```python
from build123d import *

# Parameters (mm, degrees)
SKETCH2_R           = 75
SKETCH2_R_2         = 59
SKETCH2_R_3         = 46.992946112
BOSS_EXTRUDE1_DEPTH = 6
SKETCH4_R           = 2.5
CUT_EXTRUDE1_DEPTH  = 8
SKETCH5_R           = 1.9
CUT_EXTRUDE2_DEPTH  = 8
SKETCH8_R           = 25
CUT_EXTRUDE4_DEPTH  = 2


with BuildPart() as part:
    # Sketch1 → Revolve1 (revolve)
    with BuildSketch(Plane(origin=(0, 0, 0), x_dir=(-1, 0, 0), z_dir=(0, 0, -1)), mode=Mode.PRIVATE) as revolve1_sk:
        with BuildLine():
            Line((-59, 0.8724), (-47, 0.8724))
            ThreePointArc((-47, 0.8724), (-46.292893219, 1.165293219), (-46, 1.8724))
            Line((-46, 1.8724), (-46, 5.8724))
            Line((-46, 5.8724), (-47, 6.8724))
            Line((-47, 6.8724), (-49.4043, 6.8724))
            ThreePointArc((-49.4043, 6.8724), (-52.5, 5.8405), (-55.5957, 6.8724))
            Line((-55.5957, 6.8724), (-59, 6.8724))
            Line((-59, 6.8724), (-60, 5.8724))
            Line((-60, 5.8724), (-60, 1.8724))
            ThreePointArc((-60, 1.8724), (-59.707106781, 1.165293219), (-59, 0.8724))
        make_face()
    revolve(revolve1_sk.sketch.rotate(Axis((0, 0, 0), (0, 1, 0)), 270), axis=Axis((0, 0, 0), (0, 1, 0)))

    # Sketch2 → Boss-Extrude1 (add)
    # profile 1 of 2: a face of its own
    with BuildSketch(Plane.XZ.offset(-0.8724)):
        with Locations(Location((0, 0, 0), (0, 0, 270))):
            Circle(SKETCH2_R)
        Circle(SKETCH2_R_2, mode=Mode.SUBTRACT)
    # profile 2 of 2: a face of its own
    with BuildSketch(Plane.XZ.offset(-0.8724)):
        with Locations(Location((0, 0, 0), (0, 0, 270))):
            Circle(SKETCH2_R_3)
    extrude(amount=-BOSS_EXTRUDE1_DEPTH)

    # Sketch4 → Cut-Extrude1 (cut)
    with BuildSketch(Plane.XZ.offset(-0.8724)):
        with Locations(Location((0, 0, 0), (0, 0, 270))):
            Circle(SKETCH4_R)
    extrude(amount=-CUT_EXTRUDE1_DEPTH, mode=Mode.SUBTRACT)

    # Sketch5 → Cut-Extrude2 (cut)
    with BuildSketch(Plane.XZ.offset(-0.8724)):
        with Locations(Location((0, 17.5, 0), (0, 0, 270))):
            Circle(SKETCH5_R)
        with Locations(Location((17.5, 0, 0), (0, 0, 270))):
            Circle(SKETCH5_R)
        with Locations(Location((0, -17.5, 0), (0, 0, 270))):
            Circle(SKETCH5_R)
        with Locations(Location((-17.5, 0, 0), (0, 0, 270))):
            Circle(SKETCH5_R)
    extrude(amount=-CUT_EXTRUDE2_DEPTH, mode=Mode.SUBTRACT)

    # Sketch8 → Cut-Extrude4 (cut)
    with BuildSketch(Plane(origin=(0, 6.8724, 0), x_dir=(1, 0, 0), z_dir=(0, 1, 0))):
        with Locations(Location((0, 0, 0), (0, 0, 270))):
            Circle(SKETCH8_R)
    extrude(amount=-CUT_EXTRUDE4_DEPTH, mode=Mode.SUBTRACT)


solid = part.part
```
Model file for the job. Use its own axes, mm. A direction names the side the tool comes from. Coordinates: 2 decimals unless noted, no trailing zeros. Order: outer loops, then holes, each group sorted by start corner. A loop starts at its lowest first (then second) coordinate and runs counter-clockwise, first axis right, second up. Notation, with made-up numbers: (-29.5, 51) -> (-21.5, 51) arc R15 cw to (-21.5, 63) -> close; hole circle Ø6 at (42.5, 21.25). An arc over 180 degrees is marked (long way). Answer as a JSON object with one key per item and string values. Group by question number.
1) Drill centre lines: L1, parallel to X at y = 2, z = 0; L2, parallel to X at y = 5.65, z = 0; L3, parallel to Z at x = -16, y = 6.75. Where is each one in solid material? Low to high.
2) Flat gauge pins, fed straight in: pin 1 (6 mm diameter, centred on x = 17.5, z = 0, fed in from -Y); pin 2 (1 mm diameter, centred on x = -46.5, y = 1.5, fed in from -Z); pin 3 (6 mm diameter, centred on x = 0, z = 17.5, fed in from +Y); pin 4 (1.5 mm diameter, centred on x = -51.5, z = 2.5, fed in from +Y). Where does each tip first touch, or does it go through?
3) Cut at A-A, the plane y = 3.5. Write the cut outline in (x, z), then the cut area to 3 significant figures.
4) Cut at B-B, the plane z = 0. Count the separate pieces of the cut face and the enclosed holes in it, then the cut area to 3 significant figures.
5) Which spindle directions (+Z, -Z, +X, -X, +Y, -Y) get a long thin tool onto all of the face, cutting with end or side? Do faces 4 (the face through (7.509, 5.886, 23.846)), 5 (the face through (-32.3, 0.872, 34.4)). Say none if no direction does.
6) Cut at C-C, the plane z = -61. Write the cut outline in (x, y).
7) Cut at D-D, the plane x = 62.5. Write the cut outline in (y, z), then the cut area to 3 significant figures.
8) Pull direction X, two halves, no side cores. Call faces 1 (the face through (-2.44, 2.84, 0.54)), 2 (the face through (-45.636, 3.83, 59.517)), 3 (the face through (-20, 6.872, -20)): +X half, -X half, draft (parallel to the pull), parting line (faces both ways), or undercut.
Check values:
{
 "1": {"L1": "x = -75 to -19.4, -15.6 to -2.5, 2.5 to 15.6, 19.4 to 75", "L2": "x = -75 to -25, 25 to 75", "L3": "z = -73.27 to -53.07, -46.92 to -19.21, 19.21 to 46.92, 53.07 to 73.27"},
 "2": {"pin 1": "stops at y = 0.87", "pin 2": "stops at z = -59.24", "pin 3": "stops at y = 4.87", "pin 4": "stops at y = 6.12"},
 "3": {"outline": "circle Ø150 at (0, 0); hole circle Ø3.8 at (-17.5, 0); hole circle Ø5 at (0, 0); hole circle Ø3.8 at (0, -17.5); hole circle Ø3.8 at (0, 17.5); hole circle Ø3.8 at (17.5, 0)", "area": "17,600 mm²"},
 "4": {"separate pieces": "4", "enclosed holes": "0", "area": "741 mm²"},
 "5": {"face 4": "+Y", "face 5": "+Z, -Z, +X, -X, -Y"},
 "6": {"outline": "(-43.63, 0.87) -> (43.63, 0.87) -> (43.63, 6.87) -> (-43.63, 6.87) -> close"},
 "7": {"outline": "(0.87, -41.46) -> (6.87, -41.46) -> (6.87, 41.46) -> (0.87, 41.46) -> close", "area": "497 mm²"},
 "8": {"face 1": "undercut", "face 2": "parting line", "face 3": "draft"}
}
